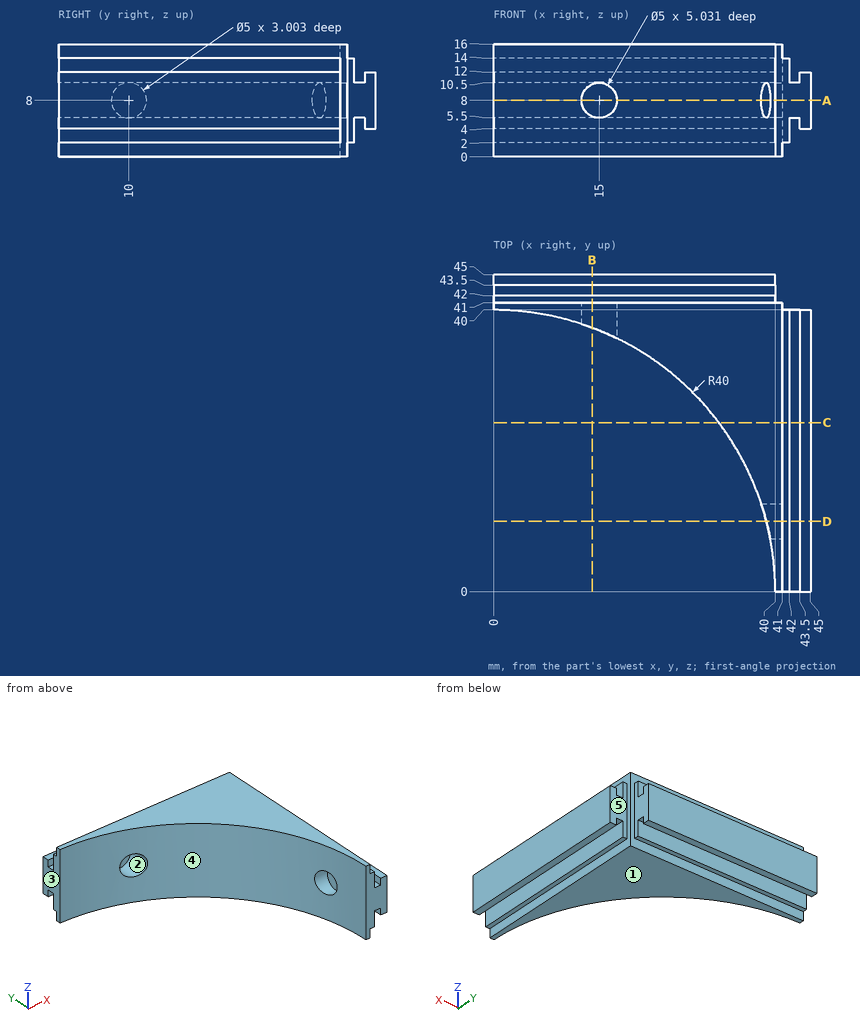
Design review of the part shown in the three views and the two pictorial views. Dimensions are in mm from the part's minimum x, y and z. A direction names the side the tool comes from. Round coordinates to 2 decimals unless told otherwise and drop trailing zeros. Write each loop counter-clockwise with the first axis right and the second up, starting at its lowest first coordinate (ties: lowest second). Pieces come first, ordered by that corner, then holes. Notation, with made-up numbers: (48.25, -7) -> (82.25, -7) arc R22 cw to (82.25, 12) -> close; hole circle Ø11 at (40.25, -20.5). An arc over 180 degrees is marked (long way). Answer as a JSON object with one key per item and string values.
1. We need section B-B on x = 14. State the section outline as (y, z) points.
Results found:
{"outline": "(37.47, 0) -> (41, 0) -> (41, 2) -> (42, 2) -> (42, 5.5) -> (43.5, 5.5) -> (43.5, 4) -> (45, 4) -> (45, 12) -> (43.5, 12) -> (43.5, 10.5) -> (42, 10.5) -> (42, 14) -> (41, 14) -> (41, 16) -> (37.47, 16) -> (37.47, 10.29) -> (41, 10.29) -> (41, 5.71) -> (37.47, 5.71) -> close"}
2. We need section A-A on z = 8. State the section outline as (x, y) points.
Results found:
{"outline": "(0, 40) arc R40 cw to (12.5, 38) -> (12.5, 41) -> (17.5, 41) -> (17.5, 35.97) arc R40 cw to (38, 12.5) -> (41, 12.5) -> (41, 7.5) -> (39.29, 7.5) arc R40 cw to (40, 0) -> (45, 0) -> (45, 40) -> (41, 40) -> (41, 41) -> (40, 41) -> (40, 45) -> (0, 45) -> close"}
3. The part is to be moulded in two halves that separate along Z. For the marked faces 1, 2 and 3, say which applies: pulls with the +Z half, pulls with the -Z half, needs draft (parallel to the pull), parting line crosses it, or undercut.
Results found:
{"face 1": "pulls with the -Z half", "face 2": "undercut", "face 3": "needs draft"}
4. Clearance check with flat-ended pins moving along their axes: pin 1 (1.6 mm diameter, centred on y = 16.5, z = 5, fed in from -X) (1 decimal); pin 2 (0.5 mm diameter, centred on x = 23.5, y = 41.5, fed in from +Z); pin 3 (1.8 mm diameter, centred on x = 20.5, z = 3, fed in from +Y). State where each tip first meets the part, or that it passes through.
Results found:
{"pin 1": "stops at x = 36.1", "pin 2": "stops at z = 14", "pin 3": "stops at y = 42"}
5. We need section C-C on y = 24. State the section outline as (x, z) points.
Results found:
{"outline": "(32, 0) -> (41, 0) -> (41, 2) -> (42, 2) -> (42, 5.5) -> (43.5, 5.5) -> (43.5, 4) -> (45, 4) -> (45, 12) -> (43.5, 12) -> (43.5, 10.5) -> (42, 10.5) -> (42, 14) -> (41, 14) -> (41, 16) -> (32, 16) -> close"}
6. To check wall thickness, follow line 1 along Y through (x, z) = (40.2, 8); line 2 along Z through (x, y) = (15, 39.85); line 3 along Y through (x, z) = (23, 11.25) (1 decimal). State the ranges of each line that lie inside material, in increasing order.
Results found:
{"line 1": "y = 0 to 7.5, 12.5 to 41", "line 2": "z = 0 to 5.5, 10.5 to 16", "line 3": "y = 32.7 to 42, 43.5 to 45"}
7. We need section D-D on y = 10. State the section outline as (x, z) points.
Results found:
{"outline": "(38.73, 0) -> (41, 0) -> (41, 2) -> (42, 2) -> (42, 5.5) -> (43.5, 5.5) -> (43.5, 4) -> (45, 4) -> (45, 12) -> (43.5, 12) -> (43.5, 10.5) -> (42, 10.5) -> (42, 14) -> (41, 14) -> (41, 16) -> (38.73, 16) -> (38.73, 10.5) -> (41, 10.5) -> (41, 5.5) -> (38.73, 5.5) -> close"}
8. Machinability: for the marked faces 4 and 5, which of the approach directions +Z, -Z, +X, -X, +Y, -Y give a long, thin tool a straight path to every point of the face, cutting with its end or side? Answer none if there is none.
Results found:
{"face 4": "+Z, -Z, -X, -Y", "face 5": "+Z, -Z, +X, +Y"}
